```python
from build123d import *

# Parameters (mm, degrees)
SKETCH1_R          = 25
BASE_FLANGE1_DEPTH = 10
FILLET1_R          = 3
CHAMFER1_SIZE      = 3


# Sheet-metal steps are written as plain solids
with BuildPart() as part:
    # Sketch1 → Base-Flange1 (new body)
    with BuildSketch(Plane(origin=(0, 0, 0), x_dir=(0, 0, -1), z_dir=(1, 0, 0))):
        with BuildLine():
            Line((-80, -46), (80, -46))
            Line((80, -46), (80, -26))
            Line((80, -26), (34.645612429, 28.717269011))
            ThreePointArc((34.645612429, 28.717269011), (0, 45), (-34.645612429, 28.717269011))
            Line((-34.645612429, 28.717269011), (-80, -26))
            Line((-80, -26), (-80, -46))
        make_face()
        Circle(SKETCH1_R, mode=Mode.SUBTRACT)
    extrude(amount=-BASE_FLANGE1_DEPTH)

    # Fillet1
    fillet1_edges = [part.edges().sort_by_distance(p)[0] for p in [
        (-10, 0, 25),
        (0, 0, 25),
    ]]
    fillet(fillet1_edges, radius=FILLET1_R)

    # Chamfer1
    chamfer1_edges = [part.edges().sort_by_distance(p)[0] for p in [
        (-10, -46, 0),
        (0, -46, 0),
    ]]
    chamfer(chamfer1_edges, length=CHAMFER1_SIZE)


solid = part.part
```
Build history of the part. All positions in model axes, mm. Round coordinates to 2 decimals unless told otherwise and drop trailing zeros. Order: outer loops, then holes, each group sorted by start corner. A loop starts at its lowest first (then second) coordinate and runs counter-clockwise, first axis right, second up. Notation, with made-up numbers: (6.25, -26) -> (20.25, -26) arc R28 cw to (20.25, -1) -> close; hole circle Ø4 at (33, 57). An arc over 180 degrees is marked (long way). Answer in a Markdown table with one row per item.
1) Band-saw the part on D-D on z = -54.5. Give the cut face in (x, y).
Values:
| item | result |
|---|---|
| outline | (-10, -43) -> (-7, -46) -> (-3, -46) -> (0, -43) -> (0, 4.76) -> (-10, 4.76) -> close |
2) Band-saw the part on A-A on z = 0. Give the cut face in (x, y), and give its area (3 significant figures).
Values:
| item | result |
|---|---|
| outline | (-10, -43) -> (-7, -46) -> (-3, -46) -> (0, -43) -> (0, -28) arc R3 ccw to (-3, -25) -> (-7, -25) arc R3 ccw to (-10, -28) -> close; (-10, 28) arc R3 ccw to (-7, 25) -> (-3, 25) arc R3 ccw to (0, 28) -> (0, 45) -> (-10, 45) -> close |
| area | 393 mm2 |
3) Band-saw the part on B-B on y = 0. Give the cut face in (x, z).
Values:
| item | result |
|---|---|
| outline | (-10, -58.45) -> (0, -58.45) -> (0, -28) arc R3 ccw to (-3, -25) -> (-7, -25) arc R3 ccw to (-10, -28) -> close; (-10, 28) arc R3 ccw to (-7, 25) -> (-3, 25) arc R3 ccw to (0, 28) -> (0, 58.45) -> (-10, 58.45) -> close |
4) Mould opens along Y. For faces 1 (the flat face through (-5, -36, 80)), 2 (the flat face through (-4.93, 1.742, 57.005)), 3 (the flat face through (-8, -45, 1)), 4 (the cylindrical face through (-4.972, 7.509, -23.846)) say: released by +Y, released by -Y, zero draft, split by the parting line, or undercut.
Values:
| item | result |
|---|---|
| face 1 | zero draft |
| face 2 | released by +Y |
| face 3 | released by -Y |
| face 4 | undercut |
5) Pin check, flat tip, straight feed: P1, Ø4, axis at x = -8.5, y = -22.5, coming from the +Z side. Stop position of the tip, or through.
Values:
| item | result |
|---|---|
| P1 | z = 78.76 |
6) Band-saw the part on C-C on z = 44. Give the cut face in (x, y).
Values:
| item | result |
|---|---|
| outline | (-10, -43) -> (-7, -46) -> (-3, -46) -> (0, -43) -> (0, 17.43) -> (-10, 17.43) -> close |
7) Wall check: L1, parallel to Y at x = -4.5, z = 0; L2, parallel to Y at x = -3, z = -12; L3, parallel to Z at x = -5.25, y = 20. Give the ranges that are in metal, low to high.
Values:
| item | result |
|---|---|
| L1 | -46 to -25, 25 to 45 |
| L2 | -46 to -21.93, 21.93 to 43.37 |
| L3 | -41.87 to -15, 15 to 41.87 |
